Check sheet for the modelled part. Datum: model origin and axes. Units: mm. Coordinates: 2 decimals unless noted, no trailing zeros. One line per item, written item: value. Start each with the question number.
1) Draft check along X on faces 1 (the flat face through (131, 29, -21)), 2 (the flat face through (104.267, 37, -20)), 3 (the cylindrical face through (148.633, 85.773, -19.521)), 4 (the cylindrical face through (171.86, 8.85, -19.52)). Enter one of: +X half, -X half, draft (parallel to the pull), parting line (faces both ways), or undercut.
2) Gauge pin test, flat ends, axial feed: P1, Ø4, axis at x = 170.52, y = 9.4, coming from the -Z side; P2, Ø1, axis at x = 123.5, z = -19, coming from the -Y side. Record the tip position at first contact, or that the pin passes through.
3) Scan lines: line 1 along Y through (x, z) = (170, -19.1); line 2 along X through (y, z) = (86.5, -19.15); line 3 along X through (y, z) = (19, -19). Record each from-to range of solid material in increasing order. Write a range as [from, to].
4) Sectioned sample at A-A on z = -18.9. Give the number of separate pieces and of enclosed holes in the cut face, plus the area to 3 significant figures.
```python
from build123d import *

# Parameters (mm, degrees)
PAD011_DEPTH    = 3
SKETCH046_R     = 1.45
POCKET014_DEPTH = 27
FILLET009_R     = 1.5
FILLET017_R     = 0.5


with BuildPart() as part:
    # Sketch035 → Pad011 (new body)
    with BuildSketch(Plane.XY):
        with BuildLine():
            add(Edge.make_bspline(
                [(104.266667, -21.941284), (120.21302, -25.349195), (134.610356, -29.830731), (153.231854, -38.154949)],
                knots=[0, 0, 0, 0, 1, 1, 1, 1], degree=3))
            Line((153.231854, -38.154949), (175.310198, 11.234895))
            add(Edge.make_bspline(
                [(150.875, 88.9625), (150.875, 42.8625), (150.875, 22.157965), (175.310198, 11.234895)],
                knots=[0, 0, 0, 0, 1, 1, 1, 1], degree=3))
            add(Edge.make_bspline(
                [(104.266667, 94.924515), (121.368889, 89.186974), (138.406555, 89.068954), (150.875, 88.9625)],
                knots=[0, 0, 0, 0, 1, 1, 1, 1], degree=3))
            Line((104.266667, 94.924515), (104.266667, -21.941284))
        make_face()
    extrude(amount=PAD011_DEPTH)

    # Sketch046 → Pocket014 (cut)
    with BuildSketch(Plane.XY):
        with Locations((-4.375, -4.375)):
            Circle(SKETCH046_R)
        with Locations((-4.375, 80.575)):
            Circle(SKETCH046_R)
        with Locations((151.401832, -33.366184)):
            Circle(SKETCH046_R)
        with Locations((170.521433, 9.404873)):
            Circle(SKETCH046_R)
        with Locations((147.25, 85.3375)):
            Circle(SKETCH046_R)
        with Locations((43.25, -13.9)):
            Circle(SKETCH046_R)
        with Locations((57.15, 92.085)):
            Circle(SKETCH046_R)
        with Locations((95.25, 92.085)):
            Circle(SKETCH046_R)
        with Locations((95.25, -13.9)):
            Circle(SKETCH046_R)
    extrude(amount=POCKET014_DEPTH, mode=Mode.SUBTRACT)

    # Fillet009
    fillet009_edges = [part.edges().sort_by_distance(p)[0] for p in [
        (153.231854, -38.154949, 1.5),
        (175.310198, 11.234895, 1.5),
        (150.875, 88.9625, 1.5),
    ]]
    fillet(fillet009_edges, radius=FILLET009_R)

    # Fillet017
    fillet017_edges = [part.edges().sort_by_distance(p)[0] for p in [
        (104.266667, 94.924515, 1.5),
        (104.266667, -21.941284, 1.5),
    ]]
    fillet(fillet017_edges, radius=FILLET017_R)


with BuildPart() as part_1:
    # Body010 placement: moved
    add(part.part.moved(Location((0, 0, -21))))


solid = part_1.part
```
Answers:
1. face 1: draft
1. face 2: -X half
1. face 3: undercut
1. face 4: undercut
2. P1: stops at z = -21
2. P2: stops at y = -27.02
3. line 1: y = [-0.64, 8.05], [10.76, 13.99]
3. line 2: x = [104.27, 146.38], [148.12, 150.88]
3. line 3: x = [104.27, 163.47]
4. separate pieces: 1
4. enclosed holes: 3
4. area: 6,490 mm2
